The listing builds one solid part. Answer for the finished solid, in the listing's coordinates (mm). A direction names the side the tool comes from. Round coordinates to 2 decimals unless told otherwise and drop trailing zeros. Order: outer loops, then holes, each group sorted by start corner. A loop starts at its lowest first (then second) coordinate and runs counter-clockwise, first axis right, second up. Notation, with made-up numbers: (27, 3) - (67, 3) arc R13 ccw to (67, 13) - close; hole circle Ø4 at (36, 83.5). An arc over 180 degrees is marked (long way). Write item = value, one per line.
from build123d import *

# Parameters (mm, degrees)
F1_DEPTH = 35
F2_R     = 4.5
F3_DEPTH = 30.87481
F4_R     = 4.5
F5_DEPTH = 35.101


with BuildPart() as f1:
    # F0 (on Right) → F1 (new body, symmetric)
    with BuildSketch(Plane.YZ):
        Polygon((-1.12619, -26.1), (-18.62619, -26.1), (-25.12619, -32.6), (-25.12619, -33.6), (-23.62619, -35.1), (30.87381, -35.1), (30.87381, 19.4), (29.37381, 20.9), (28.37381, 20.9), (21.87381, 14.4), (21.87381, -3.1), align=None)
    extrude(amount=F1_DEPTH, both=True)

    # F2 (on Front) → F3 (cut, through all)
    with BuildSketch(Plane.XZ):
        with Locations((-19.999945, 5.9)):
            Circle(F2_R)
        with Locations((20.000055, 5.9)):
            Circle(F2_R)
    extrude(amount=-F3_DEPTH, mode=Mode.SUBTRACT)

    # F4 (on Top) → F5 (cut, through all)
    with BuildSketch(Plane.XY):
        with Locations((-19.999975, -10.126112)):
            Circle(F4_R)
        with Locations((20.000025, -10.126112)):
            Circle(F4_R)
    extrude(amount=-F5_DEPTH, mode=Mode.SUBTRACT)


solid = f1.part
Q1. For faces 1 (the face through (0, 3, -35.1)), 2 (the face through (0, -10, -26.1)), determine the directions among +Z, -Z, +X, -X, +Y, -Y from which every point of the face is accessible in a straight line to the end or side of a thin tool.
Model answer:
face_1 = -Z, +X, -X, +Y, -Y
face_2 = +Z, +X, -X, -Y
Q2. Section D-D on y = 6 is taken. Determine the outline of the cut face in (x, z).
Model answer:
outline = (-35, -35.1) - (35, -35.1) - (35, -18.97) - (-35, -18.97) - close
Q3. Flat-ended cylindrical pins translate along their axes: P1, Ø19, axis at x = 12, y = -8.5, coming from the +Z side; P2, Ø6, axis at x = -15.5, y = -15.5, coming from the +Z side; P3, Ø10, axis at x = -8, z = 13, coming from the -Y side. Find the tip coordinate at first contact, or state that the pin passes through.
Model answer:
P1 = -23.97
P2 = -26.1
P3 = 21.87
Q4. Section C-C on x = 5.5 is taken. Determine the outline of the cut face in (y, z), then the cut area to 3 significant figures.
Model answer:
outline = (-25.13, -33.6) - (-23.63, -35.1) - (30.87, -35.1) - (30.87, 19.4) - (29.37, 20.9) - (28.37, 20.9) - (21.87, 14.4) - (21.87, -3.1) - (-1.13, -26.1) - (-18.63, -26.1) - (-25.13, -32.6) - close
area = 1,150 mm^2
Q5. Find the intervals of material crossed by line 1 (Z direction, x = -2.5, y = -18); line 2 (Y direction, x = -4, z = 7); line 3 (X direction, y = 27, z = 5), in increasing order. Write a range as from..to.
Model answer:
line_1 = -35.1..-26.1
line_2 = 21.87..30.87
line_3 = -35..-24.41, -15.59..15.59, 24.41..35
Q6. Section B-B on x = -20.5 is taken. Determine the outline of the cut face in (y, z), then the cut area to 3 significant figures.
Model answer:
outline = (-25.13, -33.6) - (-23.63, -35.1) - (-14.6, -35.1) - (-14.6, -26.1) - (-18.63, -26.1) - (-25.13, -32.6) - close; (-5.65, -35.1) - (30.87, -35.1) - (30.87, 1.43) - (21.87, 1.43) - (21.87, -3.1) - (-1.13, -26.1) - (-5.65, -26.1) - close; (21.87, 10.37) - (30.87, 10.37) - (30.87, 19.4) - (29.37, 20.9) - (28.37, 20.9) - (21.87, 14.4) - close
area = 986 mm^2
Q7. Determine the mould class of faces 3 (the face through (-35, 13, -17)), 4 (the face through (0, 21.874, 6)), 5 (the face through (-17.923, -14.118, -30.537)) for opening direction X: released by +X, released by -X, zero draft, split by the parting line, or undercut.
Model answer:
face_3 = released by -X
face_4 = zero draft
face_5 = undercut
Q8. Section A-A on z = 5.9 is taken. Determine the outline of the cut face in (x, y).
Model answer:
outline = (-35, 21.87) - (-24.5, 21.87) - (-24.5, 30.87) - (-35, 30.87) - close; (-15.5, 21.87) - (15.5, 21.87) - (15.5, 30.87) - (-15.5, 30.87) - close; (24.5, 21.87) - (35, 21.87) - (35, 30.87) - (24.5, 30.87) - close
